Autodesk Inventor part; units mm, degrees
ref_plane "YZ Plane" through (0, 0, 0) normal (1, 0, 0) x (0, 1, 0)
ref_plane "XZ Plane" through (0, 0, 0) normal (0, 1, 0) x (-1, 0, 0)
ref_plane "XY Plane" through (0, 0, 0) normal (0, 0, 1) x (1, 0, 0)
sketch "Sketch1" plane through (0, 0, 0) normal (0, 1, 0) x (-1, 0, 0)
  line L0 (5.5664, 6.3616) -> (-16.4336, 6.3616)
  line L1 (-16.4336, 6.3616) -> (-16.4336, -7.8384)
  line L2 (-16.4336, -7.8384) -> (5.5664, -7.8384)
  line L3 (5.5664, -7.8384) -> (5.5664, 6.3616)
  point P0 (0, 0)
  dimension "d2" = 14.2
  dimension "d3" = 22
extrude "Extrusion1" add sketch "Sketch1" along normal blind 10.4
sketch "Sketch2" plane through (0, 10.4, 0) normal (0, 1, 0) x (1, 0, 0)
  line L0 (-5.5664, -6.3616) -> (16.4336, -6.3616)
  line L1 (16.4336, -6.3616) -> (16.4336, 7.8384)
  line L2 (16.4336, 7.8384) -> (-5.5664, 7.8384)
  line L3 (-5.5664, 7.8384) -> (-5.5664, -6.3616)
  line L4 (-5.5664, -6.3616) -> (16.4336, -6.3616)
  line L5 (-4.3664, -6.3616) -> (-4.3664, 7.8384)
  line L6 (-5.5664, 7.8384) -> (-5.5664, -6.3616)
  line L7 (-5.5664, 7.2384) -> (16.4336, 7.2384)
  line L8 (16.4336, -6.3616) -> (16.4336, 7.8384)
  circle A0 centre (-2.5164, 5.3884) radius 1.85
  circle A1 centre (-2.5164, 5.3884) radius 1.7
  point P0 (0, 0)
  point P1 (5.4336, 7.2384)
  dimension "d4" = 1.2
  dimension "d5" = 0.6
  dimension "d6" = 3.7
  dimension "d8" = 3.4
extrude "Extrusion2" cut sketch "Sketch2" against normal through all draft -2 contours A1
fillet "Fillet1" radius 0.5 4 edges at (16.4336, 5.2, 6.3616) (16.4336, 5.2, -7.8384) (-5.5664, 5.2, -7.8384) (-5.5664, 5.2, 6.3616)
chamfer "Chamfer1" distance 0.5 angle 45 1 edges at (-4.2164, 10.4, -5.3884)
properties part number "podpora_imu"
CAD build for the part. Positions are in the model's coordinates, mm. Round coordinates to 2 decimals unless told otherwise and drop trailing zeros. Write each loop counter-clockwise with the first axis right and the second up, starting at its lowest first coordinate (ties: lowest second). Pieces come first, ordered by that corner, then holes. Notation, with made-up numbers: M -17,4.5 L -9,4.5 A14 ccw -9,28.5 Z; hole C -9,75.25 d1. An arc over 180 degrees is marked long. Put each result on its own line as item: value. Start each with the question number.
1) Saw through at A-A, the plane y = 4.5. Write the cut outline in (x, z).
2) Saw through at B-B, the plane y = 6. Write the cut outline in (x, z).
3) Drill centre lines: probe 1 along X at (y, z) = (8.25, -4); probe 2 along X at (y, z) = (1, -4.25); probe 3 along Y at (x, z) = (-3, -3.5). Where is each one in solid material? Low to high. Write a range as [from, to].
4) Pull direction Z, two halves, no side cores. Call faces 1 (the flat face through (6, 0, -1)), 2 (the conical face through (-1.819, 5.019, -4.047)), 3 (the flat face through (6, 5, -7.838)): pulls with the +Z half, pulls with the -Z half, needs draft (parallel to the pull), parting line crosses it, or undercut.
Resolved:
1. outline: M -5.57,-7.34 A0.5 ccw -5.07,-7.84 L 15.93,-7.84 A0.5 ccw 16.43,-7.34 L 16.43,5.86 A0.5 ccw 15.93,6.36 L -5.07,6.36 A0.5 ccw -5.57,5.86 Z; hole C -2.52,-5.39 d2.99
2. outline: M -5.57,-7.34 A0.5 ccw -5.07,-7.84 L 15.93,-7.84 A0.5 ccw 16.43,-7.34 L 16.43,5.86 A0.5 ccw 15.93,6.36 L -5.07,6.36 A0.5 ccw -5.57,5.86 Z; hole C -2.52,-5.39 d3.09
3. probe 1: [-5.57, -3.36], [-1.67, 16.43]
3. probe 2: [-5.57, -3.28], [-1.75, 16.43]
3. probe 3: [0, 10.16]
4. face 1: needs draft
4. face 2: undercut
4. face 3: pulls with the -Z half
